Work out the finished part from the listing and answer in its coordinate system (mm). A direction names the side the tool comes from. Give positions to 0.01 mm unless a question says otherwise; leave off trailing zeros. Order: outer loops, then holes, each group sorted by start corner. A loop starts at its lowest first (then second) coordinate and runs counter-clockwise, first axis right, second up. Notation, with made-up numbers: (4, -32) - (10, -32) arc R20 cw to (10, 2) - close; hole circle Ø3 at (-18.75, 14). An arc over 180 degrees is marked (long way). Write each question's results on one line, items separated by ' | '.
Autodesk Inventor part; units mm, degrees
ref_plane "YZ Plane" through (0, 0, 0) normal (1, 0, 0) x (0, 1, 0)
ref_plane "XZ Plane" through (0, 0, 0) normal (0, 1, 0) x (-1, 0, 0)
ref_plane "XY Plane" through (0, 0, 0) normal (0, 0, 1) x (1, 0, 0)
sketch "Sketch1" plane through (0, 0, 0) normal (1, 0, 0) x (0, 1, 0)
  line L0 (7, 7) -> (-7, 7)
  line L1 (-7, 7) -> (-7, -7)
  line L2 (-7, -7) -> (7, -7)
  line L3 (7, -7) -> (7, 7)
  line L4 (7, 7) -> (-7, -7) construction
  line L5 (-7, 7) -> (7, -7) construction
  line L6 (6, 8) -> (-6, 8)
  line L7 (-8, 6) -> (-8, -6)
  line L8 (-6, -8) -> (6, -8)
  line L9 (8, -6) -> (8, 6)
  line L10 (8, 8) -> (-8, -8) construction
  line L11 (-8, 8) -> (8, -8) construction
  arc A0 (8, 6) -> (6, 8) centre (6, 6) ccw
  arc A1 (-6, 8) -> (-8, 6) centre (-6, 6) ccw
  arc A2 (-8, -6) -> (-6, -8) centre (-6, -6) ccw
  arc A3 (6, -8) -> (8, -6) centre (6, -6) ccw
  point P0 (0, 0)
  dimension "d0" = 14
  dimension "d1" = 14
  dimension "d2" = 16
  dimension "d3" = 16
  dimension "d4" = 2
extrude "Extrusion1" add sketch "Sketch1" along normal blind 100
properties part number "suspension2chassis"
1. A cutting plane is placed at A-A, the plane y = 2.25. Write down the section's boundary in (x, z), then the cut area to 3 significant figures.
Answer list:
outline: (0, -8) - (100, -8) - (100, -7) - (0, -7) - close; (0, 7) - (100, 7) - (100, 8) - (0, 8) - close | area: 200 mm^2
2. Straight lines are drawn through the part: line 1 (Z direction, x = 42, y = -3.5); line 2 (Y direction, x = 74.5, z = 6.5). For each, find the intervals that lie inside material, in ascending order. Write a range as [from, to].
Answer list:
line 1: [-8, -7], [7, 8] | line 2: [-7.94, -7], [7, 7.94]
3. Determine the mould class of faces 1 (the face through (49, -7, 0)), 2 (the face through (0, -7.15, 0.63)), 3 (the face through (49.3, 7.43, -7.4)) for opening direction Y: +Y half, -Y half, draft (parallel to the pull), parting line (faces both ways), or undercut.
Answer list:
face 1: undercut | face 2: draft | face 3: +Y half
4. A cutting plane is placed at C-C, the plane x = 24. Write down the section's boundary in (y, z).
Answer list:
outline: (-8, -6) arc R2 ccw to (-6, -8) - (6, -8) arc R2 ccw to (8, -6) - (8, 6) arc R2 ccw to (6, 8) - (-6, 8) arc R2 ccw to (-8, 6) - close; hole (-7, -7) - (7, -7) - (7, 7) - (-7, 7) - close
5. A tool of negligible diameter and unlimited length cuts with its end or side. For faces 4 (the face through (49, 0, 7)), 5 (the face through (49, 0, -8)), from which of +Z, -Z, +X, -X, +Y, -Y can it reach the whole face along a straight path? Write none if from no direction.
Answer list:
face 4: +X, -X | face 5: -Z, +X, -X, +Y, -Y
